Design review of the part built by this model. Coordinates are the model's own, in mm. A direction names the side the tool comes from. Coordinates: 2 decimals unless noted, no trailing zeros. Write each loop counter-clockwise with the first axis right and the second up, starting at its lowest first coordinate (ties: lowest second). Pieces come first, ordered by that corner, then holes. Notation, with made-up numbers: (86.5, -21.5) -> (126.5, -21.5) arc R8 cw to (126.5, -15.5) -> close; hole circle Ø5 at (47.25, 82.5). An arc over 180 degrees is marked (long way). One line per question, with ' | ' between items. Start each with the question number.
Q1. For P1, Ø2.5, axis at x = 26.5, y = -34.5, coming from the -Z side, flat-tipped, find the tip position at first contact; note if it passes through.
Q2. Add section B-B on x = -7. State the section outline as (y, z) points (3 decimals), and give its area (3 significant figures).
Q3. Wall thickness on probe 1 along Y at (x, z) = (54, 5.4) (1 decimal); probe 2 along Y at (x, z) = (27, 2.1) (1 decimal); probe 3 along Y at (x, z) = (-22.5, 3.6) (3 decimals): over which ranges is each line inside the solid? List them lowest first.
Q4. For faces 1 (the cylindrical face through (27.49, 59.83, 1.97)), 2 (the cylindrical face through (-53.031, -37.576, 5.191)), 3 (the flat face through (18, -18, 2.35)), list the 3-axis set-ups (+Z, -Z, +X, -X, +Y, -Y) from which the entire face can be reached by the end or side of a thin tool; tool diameter is ignored.
Q5. Add section A-A on x = -54. Give the number of separate pieces and of enclosed holes in the cut face, and give its area (3 significant figures).
from build123d import *

# Parameters (mm, degrees)
SKETCH1_W                                    = 172
SKETCH1_H                                    = 120
BOSS_EXTRUDE1_DEPTH                          = 6.35
CBORE_FOR_M4_HEX_HEAD_CAP_SCREW1_D           = 4.2
CBORE_FOR_M4_HEX_HEAD_CAP_SCREW1_CBORE_D     = 7.6
CBORE_FOR_M4_HEX_HEAD_CAP_SCREW1_CBORE_DEPTH = 4
SKETCH4_R                                    = 17.5
CUT_EXTRUDE1_DEPTH                           = 106.053902831
CBORE_FOR_M4_HEX_HEAD_CAP_SCREW2_D           = 4.2
CBORE_FOR_M4_HEX_HEAD_CAP_SCREW2_CBORE_D     = 7.6
CBORE_FOR_M4_HEX_HEAD_CAP_SCREW2_CBORE_DEPTH = 4
SKETCH7_W                                    = 120
SKETCH7_H                                    = 25.175
CUT_EXTRUDE2_DEPTH                           = 106.053902831


with BuildPart() as part:
    # Sketch1 → Boss-Extrude1 (new body)
    with BuildSketch(Plane(origin=(0, 0, 0), x_dir=(0, 1, 0), z_dir=(0, 0, 1))):
        Rectangle(SKETCH1_W, SKETCH1_H)
    extrude(amount=BOSS_EXTRUDE1_DEPTH)

    # CBORE for M4 Hex Head Cap Screw1 (through all)
    with Locations(Plane(origin=(0, -22.5, 6.35), x_dir=(1, 0, 0), z_dir=(0, 0, 1))):
        with Locations((0, 0), (-15.909902577, 6.590097423), (-22.5, 22.5), (-15.909902577, 38.409902577), (0, 45), (15.909902577, 38.409902577), (22.5, 22.5), (15.909902577, 6.590097423)):
            CounterBoreHole(CBORE_FOR_M4_HEX_HEAD_CAP_SCREW1_D / 2, CBORE_FOR_M4_HEX_HEAD_CAP_SCREW1_CBORE_D / 2, CBORE_FOR_M4_HEX_HEAD_CAP_SCREW1_CBORE_DEPTH)

    # Sketch4 → Cut-Extrude1 (cut, through all)
    with BuildSketch(Plane.XY.offset(6.35)):
        Circle(SKETCH4_R)
    extrude(amount=-CUT_EXTRUDE1_DEPTH, mode=Mode.SUBTRACT)

    # CBORE for M4 Hex Head Cap Screw2 (through all)
    with Locations(Plane(origin=(-54, -81.2375, 0), x_dir=(-1, 0, 0), z_dir=(0, 0, -1))):
        with Locations((0, 0), (-27, 0), (-54, 0), (-81, 0), (-108, 0), (0, 45.525), (-27, 45.525), (-54, 45.525), (-81, 45.525), (-108, 45.525), (0, 137.3), (-27, 137.3), (-54, 137.3), (-81, 137.3), (-108, 137.3)):
            CounterBoreHole(CBORE_FOR_M4_HEX_HEAD_CAP_SCREW2_D / 2, CBORE_FOR_M4_HEX_HEAD_CAP_SCREW2_CBORE_D / 2, CBORE_FOR_M4_HEX_HEAD_CAP_SCREW2_CBORE_DEPTH)

    # Sketch7 → Cut-Extrude2 (cut, through all)
    with BuildSketch(Plane.XY.offset(6.35)):
        with Locations((0, 73.4125)):
            Rectangle(SKETCH7_W, SKETCH7_H)
    extrude(amount=-CUT_EXTRUDE2_DEPTH, mode=Mode.SUBTRACT)


solid = part.part
Output values:
1) P1: stops at z = 4
2) outline: (-86, 0) -> (-16.039, 0) -> (-16.039, 6.35) -> (-86, 6.35) -> close; (16.039, 0) -> (60.825, 0) -> (60.825, 6.35) -> (16.039, 6.35) -> close | area: 729 mm2
3) probe 1: y = -86 to -83.3, -79.1 to -37.8, -33.6 to 54, 58.2 to 60.8 | probe 2: y = -86 to -85, -77.4 to -39.5, -31.9 to 52.3, 59.9 to 60.8 | probe 3: y = -86 to -3.8, 3.8 to 60.825
4) face 1: -Z | face 2: +Z, -Z | face 3: +Z
5) separate pieces: 4 | enclosed holes: 0 | area: 812 mm2
